from build123d import *

# Parameters (mm, degrees)
SKETCH001_R     = 1.5
SKETCH001_R_2   = 2.65
PAD_DEPTH       = 14
SKETCH_R        = 2.65
POCKET_DEPTH    = 68.001
SKETCH002_W     = 60
SKETCH002_H     = 17
POCKET001_DEPTH = 4
SKETCH003_W     = 60
SKETCH003_H     = 17
POCKET002_DEPTH = 4
CHAMFER_SIZE    = 2
FILLET_R        = 2
FILLET001_R     = 2
SKETCH004_R     = 1.65
POCKET003_DEPTH = 10.001


with BuildPart() as part:
    # Sketch001 → Pad (new body)
    with BuildSketch(Plane.XY):
        Polygon((30, 21), (34, 21), (34, -21), (30, -21), (30, -8.5), (-30, -8.5), (-30, -21), (-34, -21), (-34, 21), (-30, 21), (-30, 8.5), (30, 8.5), align=None)
        with Locations((-14.5, 0)):
            Circle(SKETCH001_R, mode=Mode.SUBTRACT)
        with Locations((-18.5, 0)):
            Circle(SKETCH001_R, mode=Mode.SUBTRACT)
        with Locations((-25, 0)):
            Circle(SKETCH001_R_2, mode=Mode.SUBTRACT)
        with Locations((15, 0)):
            Circle(SKETCH001_R_2, mode=Mode.SUBTRACT)
    extrude(amount=PAD_DEPTH)

    # Sketch (on Face11 of Pad) → Pocket (cut, through all)
    with BuildSketch(Plane(origin=(-34, 0, 0), x_dir=(0, -1, 0), z_dir=(-1, 0, 0))):
        with Locations((-16, 7)):
            Circle(SKETCH_R)
        with Locations((16, 7)):
            Circle(SKETCH_R)
    extrude(amount=-POCKET_DEPTH, mode=Mode.SUBTRACT)

    # Sketch002 (on Face4 of Pocket) → Pocket001 (cut)
    with BuildSketch(Plane.XY.offset(14)):
        Rectangle(SKETCH002_W, SKETCH002_H)
    extrude(amount=-POCKET001_DEPTH, mode=Mode.SUBTRACT)

    # Sketch003 (on Face4 of Pocket) → Pocket002 (cut)
    with BuildSketch(Plane.XY):
        Rectangle(SKETCH003_W, SKETCH003_H)
    extrude(amount=POCKET002_DEPTH, mode=Mode.SUBTRACT)

    # Chamfer
    chamfer_edges = [part.edges().sort_by_distance(p)[0] for p in [
        (-30, 8.5, 7),
        (30, 8.5, 7),
        (30, -8.5, 7),
        (-30, -8.5, 7),
    ]]
    chamfer(chamfer_edges, length=CHAMFER_SIZE)

    # Fillet
    fillet_edges = [part.edges().sort_by_distance(p)[0] for p in [
        (32, -21, 14),
        (32, -21, 0),
        (32, 21, 14),
        (32, 21, 0),
    ]]
    fillet(fillet_edges, radius=FILLET_R)

    # Fillet001
    fillet001_edges = [part.edges().sort_by_distance(p)[0] for p in [
        (-32, 21, 14),
        (-32, 21, 0),
        (-32, -21, 14),
        (-32, -21, 0),
    ]]
    fillet(fillet001_edges, radius=FILLET001_R)

    # Sketch004 (on Face6 of Fillet001) → Pocket003 (cut, through all)
    with BuildSketch(Plane(origin=(0, 0, 4), x_dir=(1, 0, 0), z_dir=(0, 0, -1))):
        Circle(SKETCH004_R)
    extrude(amount=-POCKET003_DEPTH, mode=Mode.SUBTRACT)


solid = part.part
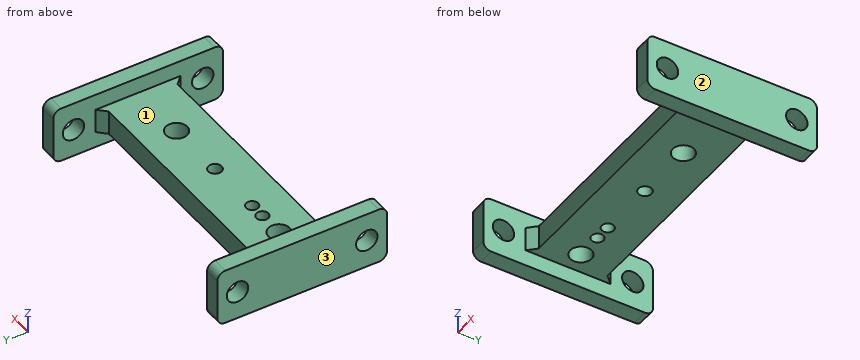
Work out the finished part from the listing and answer in its coordinate system (mm). Face numbers are marked on the shaded views. Coordinates: 2 decimals unless noted, no trailing zeros. Loops run counter-clockwise (first coordinate to the right, second up) from the corner with the lowest first, then second, coordinate; pieces in that order, holes last. Notation, with made-up numbers: M 6,77.5 L 53,77.5 A17 cw 53,86.5 Z; hole C -4.5,-14 d6. An arc over 180 degrees is marked long. Answer in a Markdown table with one row per item. Add a question column.
1. Find section D-D, the plane x = 0. Write down the section's boundary in (y, z).
2. Find section A-A, the plane y = 0. State how many separate pieces and enclosed holes the cut face has, then the cut area to 3 significant figures.
3. Find section B-B, the plane x = -25. Write down the section's boundary in (y, z), then the cut area to 3 significant figures.
4. The mould has two halves that part along X. Classify the marked faces 1, 2 and 3: pulls with the +X half, pulls with the -X half, needs draft (parallel to the pull), parting line crosses it, or undercut.
5. Find section C-C, the plane y = -16. Write down the section's boundary in (x, z).
6. Flat-ended cylindrical pins translate along their axes: P1, Ø3, axis at x = 12.5, z = 7, coming from the +Y side; P2, Ø23, axis at x = 2.5, y = -2.5, coming from the +Z side; P3, Ø23, axis at x = -3.5, y = 4.5, coming from the -Z side. Find the tip coordinate at first contact, or state that the pin passes through.
7. Consider L1, parallel to X at y = 0, z = 8.2; L2, parallel to Y at x = 0, z = 6.6; L3, parallel to X at y = 17, z = 12. Determine where each line is inside the solid, lowest interval first.
Reported:
| question | item | result |
|---|---|---|
| 1 | outline | M -8.5,4 L -1.65,4 L -1.65,10 L -8.5,10 Z; M 1.65,4 L 8.5,4 L 8.5,10 L 1.65,10 Z |
| 2 | separate pieces | 6 |
| 2 | enclosed holes | 0 |
| 2 | area | 353 mm^2 |
| 3 | outline | M -8.5,4 L -2.65,4 L -2.65,10 L -8.5,10 Z; M 2.65,4 L 8.5,4 L 8.5,10 L 2.65,10 Z |
| 3 | area | 70.2 mm^2 |
| 4 | face 1 | undercut |
| 4 | face 2 | pulls with the +X half |
| 4 | face 3 | pulls with the -X half |
| 5 | outline | M -34,0 L -30,0 L -30,4.35 L -34,4.35 Z; M -34,9.65 L -30,9.65 L -30,14 L -34,14 Z; M 30,0 L 34,0 L 34,4.35 L 30,4.35 Z; M 30,9.65 L 34,9.65 L 34,14 L 30,14 Z |
| 6 | P1 | stops at y = 8.5 |
| 6 | P2 | stops at z = 10 |
| 6 | P3 | stops at z = 4 |
| 7 | L1 | x = -34 to -27.65, -22.35 to -20, -17 to -16, -13 to -1.65, 1.65 to 12.35, 17.65 to 34 |
| 7 | L2 | y = -8.5 to -1.65, 1.65 to 8.5 |
| 7 | L3 | x = -34 to -30, 30 to 34 |
